```python
from build123d import *

# Parameters (mm, degrees)
ESQUISSE2_R             = 7
BOSS_EXTRU_2_DEPTH      = 22
ENL_V_MAT_EXTRU_1_DEPTH = 19
ESQUISSE5_R             = 5.5
ENL_V_MAT_EXTRU_2_DEPTH = 105.177732746
ENL_V_START             = -36
ENL_V_MAT_EXTRU_3_DEPTH = 24
COQUE1_START            = 3
COQUE1_DEPTH            = 19
COQUE1_START_2          = 15
COQUE1_2_OUTLINE_R      = 6.5
COQUE1_2_DEPTH          = 7
ENL_V_MAT_EXTRU_4_REACH = 106.178
ESQUISSE16_R            = 6.5
ENL_V_START_2           = -13
ENL_V_MAT_EXTRU_5_DEPTH = 13


# Read off the part's stored shape, not the designer's step: Coque1
with BuildPart() as part:
    # Esquisse2 → Boss.-Extru.2 (new, symmetric)
    with BuildSketch(Plane.XY):
        with BuildLine():
            Line((51.296980053, -19), (57, -19))
            Line((57, -19), (86, 15))
            Line((86, 15), (86, 34))
            Line((86, 34), (81, 39))
            Line((81, 39), (57, 39))
            ThreePointArc((57, 39), (48.490791592, 29.99016727), (36.246410316, 28.077357637))
            Line((36.246410316, 28.077357637), (14, 32))
            Line((14, 32), (7, 32))
            Line((7, 32), (0, 25))
            Line((0, 25), (0, 7))
            Line((0, 7), (7, 0))
            Line((7, 0), (39.575538911, 0))
            ThreePointArc((39.575538911, 0), (42.840774692, -1.213413768), (44.521177653, -4.264705882))
            ThreePointArc((44.521177653, -4.264705882), (46.858007856, -12.115672061), (51.296980053, -19))
        make_face()
        with Locations((14, 14)):
            Circle(ESQUISSE2_R, mode=Mode.SUBTRACT)
    extrude(amount=BOSS_EXTRU_2_DEPTH, both=True)

    # Esquisse4 → Enlèv. mat.-Extru.1 (cut)
    with BuildSketch(Plane.XY.offset(22)):
        Polygon((34, 32), (0, 32), (0, -19), (86, -19), (86, 0), (34, 0), align=None)
    extrude(amount=-ENL_V_MAT_EXTRU_1_DEPTH, mode=Mode.SUBTRACT)

    # Esquisse5 → Enlèv. mat.-Extru.2 (cut, through all)
    with BuildSketch(Plane.XY.offset(22)):
        with Locations((72, 25)):
            Circle(ESQUISSE5_R)
    extrude(amount=-ENL_V_MAT_EXTRU_2_DEPTH, mode=Mode.SUBTRACT)

    # Esquisse14 → Enlèv. mat.-Extru.3 (cut)
    with BuildSketch(Plane(origin=(0, 0, -22), x_dir=(-1, 0, 0), z_dir=(0, 0, -1)).offset(ENL_V_START)):
        with BuildLine():
            Line((-75.764705882, 3), (-86, 15))
            Line((-86, 15), (-86, 34))
            Line((-86, 34), (-81, 39))
            Line((-81, 39), (-57, 39))
            ThreePointArc((-57, 39), (-53.002548038, 33.285750119), (-47.224051208, 29.381745985))
            ThreePointArc((-47.224051208, 29.381745985), (-58.169717695, 12.59414375), (-75.764705882, 3))
        make_face()
    extrude(amount=ENL_V_MAT_EXTRU_3_DEPTH, mode=Mode.SUBTRACT)

    # Coque1 outline → Coque1 (cut)
    with BuildSketch(Plane.XY.offset(COQUE1_START)):
        with BuildLine():
            Line((72.744476296, 1), (73.986847747, 2.456573425))
            ThreePointArc((73.986847747, 2.456573425), (57.296143365, 12.041008897), (46.63326541, 28.064243583))
            ThreePointArc((46.63326541, 28.064243583), (41.418086005, 26.871182604), (36.072762138, 27.092549884))
            Line((36.072762138, 27.092549884), (35, 27.281706793))
            Line((35, 27.281706793), (35, 1))
            Line((35, 1), (72.744476296, 1))
        make_face()
    extrude(amount=COQUE1_DEPTH, mode=Mode.SUBTRACT)

    # Coque1 2 outline → Coque1 2 (cut)
    with BuildSketch(Plane.XY.offset(COQUE1_START_2)):
        with BuildLine():
            Line((73.986847747, 2.456573425), (85, 15.368545033))
            Line((85, 15.368545033), (85, 33.585786438))
            Line((85, 33.585786438), (80.585786438, 38))
            Line((80.585786438, 38), (57.631958739, 38))
            ThreePointArc((57.631958739, 38), (53.079347815, 31.984103338), (46.63326541, 28.064243583))
            ThreePointArc((46.63326541, 28.064243583), (57.296143365, 12.041008897), (73.986847747, 2.456573425))
        make_face()
        with Locations((72, 25)):
            Circle(COQUE1_2_OUTLINE_R, mode=Mode.SUBTRACT)
    extrude(amount=COQUE1_2_DEPTH, mode=Mode.SUBTRACT)

    # Esquisse16 → Enlèv. mat.-Extru.4 (cut, up to next)
    with BuildSketch(Plane.XY.offset(22), mode=Mode.PRIVATE) as enl_v_mat_extru_4_sk1:
        with Locations(Location((72, 25, 0), (0, 0, 180))):
            Circle(ESQUISSE16_R)
    enl_v_mat_extru_4_tool1 = extrude(enl_v_mat_extru_4_sk1.sketch, amount=-ENL_V_MAT_EXTRU_4_REACH, mode=Mode.PRIVATE) & part.part
    add(enl_v_mat_extru_4_tool1.solids().sort_by_distance((72, 25, 22))[0], mode=Mode.SUBTRACT)

    # Esquisse17 → Enlèv. mat.-Extru.5 (cut)
    with BuildSketch(Plane.XY.offset(3).offset(ENL_V_START_2)):
        with BuildLine():
            Line((72.744476296, 1), (73.986847747, 2.456573425))
            ThreePointArc((73.986847747, 2.456573425), (57.296143365, 12.041008897), (46.63326541, 28.064243583))
            ThreePointArc((46.63326541, 28.064243583), (41.418086005, 26.871182604), (36.072762138, 27.092549884))
            Line((36.072762138, 27.092549884), (35, 27.281706793))
            Line((35, 27.281706793), (35, 1))
            Line((35, 1), (72.744476296, 1))
        make_face()
    extrude(amount=ENL_V_MAT_EXTRU_5_DEPTH, mode=Mode.SUBTRACT)


solid = part.part
```
For this review, take the finished solid that the model builds, in its own axes (mm). A direction names the side the tool comes from. Round coordinates to 2 decimals unless told otherwise and drop trailing zeros. Write each loop counter-clockwise with the first axis right and the second up, starting at its lowest first coordinate (ties: lowest second). Pieces come first, ordered by that corner, then holes. Notation, with made-up numbers: (44, 80.25) - (68, 80.25) arc R24 cw to (68, 113.25) - close; hole circle Ø3 at (44, 88). An arc over 180 degrees is marked (long way). Answer as CSV lines item,"result". Start each with the question number.
(1) For line 1 (Y direction, x = 72, z = 14.4); line 2 (Z direction, x = 42, y = 11); line 3 (Y direction, x = 14, z = -9), list the stretches that pass through material, from the lowest coordinate up.
(2) Add section C-C, the plane z = -6. State the section outline as (x, y) points.
(3) Machinability: for faces 4 (the cylindrical face through (65.8, 23.05, 14.51)), 5 (the flat face through (56, -7, 3)), 6 (the flat face through (11, 32, -9)), which of the approach directions +Z, -Z, +X, -X, +Y, -Y give a long, thin tool a straight path to every point of the face, cutting with its end or side? Answer none if there is none.
(4) For pin 1 (1.5 mm diameter, centred on x = 65.5, y = 24, fed in from +Z); pin 2 (3.5 mm diameter, centred on x = 65.5, z = 19.5, fed in from -Y); pin 3 (13 mm diameter, centred on y = 12, z = 3, fed in from +X); pin 4 (10.5 mm diameter, centred on x = 72, y = 25, fed in from +Z), all flat-tipped, find the tip position at first contact; note any pin that passes through.
(5) Add section D-D, the plane x = 63. State the section outline as (y, z) points.
(6) Add section B-B, the plane y = 8. State the section outline as (x, z) points, plus the area to 3 significant figures.
(7) Add section A-A, the plane z = 9.5. State the section outline as (x, y) points, plus the area to 3 significant figures.
(8) Mouldability with a two-part tool opening along X and no side actions: class faces 1 (the cylindrical face through (57.495, 11.856, 2.325)), 2 (the flat face through (46, 28, 22)), 3 (the cylindrical face through (42.8, -1.18, -9.32)) as +X half, -X half, draft (parallel to the pull), parting line (faces both ways), or undercut.
From the geometry:
1,line 1,"y = 0 to 1, 3.1 to 18.5, 31.5 to 39"
1,line 2,"z = -22 to -10"
1,line 3,"y = 0 to 7, 21 to 32"
2,outline,"(0, 7) - (7, 0) - (39.58, 0) arc R5 cw to (44.52, -4.26) arc R29 ccw to (51.3, -19) - (57, -19) - (75.76, 3) arc R41 cw to (47.22, 29.38) arc R19.15 cw to (36.25, 28.08) - (14, 32) - (7, 32) - (0, 25) - close; hole circle Ø14 at (14, 14); hole (35, 1) - (72.74, 1) - (73.99, 2.46) arc R42 cw to (46.63, 28.06) arc R20.15 cw to (36.07, 27.09) - (35, 27.28) - close"
3,face 4,"+Z"
3,face 5,"+Z, +X, -X, -Y"
3,face 6,"+Z, -Z, -X, +Y"
4,pin 1,"stops at z = 15"
4,pin 2,"stops at y = 0"
4,pin 3,"stops at x = 68.77"
4,pin 4,"passes through"
5,outline,"(-11.97, -22) - (39, -22) - (39, -10) - (8.76, -10) - (8.76, 14) - (39, 14) - (39, 22) - (38, 22) - (38, 15) - (7.56, 15) - (7.56, -10) - (1, -10) - (1, 22) - (0, 22) - (0, 3) - (-11.97, 3) - close"
6,outline,"(0, -22) - (10.39, -22) - (10.39, 3) - (0, 3) - close; (17.61, -22) - (80.03, -22) - (80.03, -10) - (64.16, -10) - (64.16, 14) - (80.03, 14) - (80.03, 22) - (78.72, 22) - (78.72, 15) - (62.34, 15) - (62.34, -10) - (35, -10) - (35, 22) - (34, 22) - (34, 3) - (17.61, 3) - close"
6,area,"1,320 mm²"
7,outline,"(34, 0) - (73.21, 0) - (75.76, 3) arc R41 cw to (47.22, 29.38) arc R19.15 cw to (36.25, 28.08) - (34, 28.47) - close; hole (35, 1) - (72.74, 1) - (73.99, 2.46) arc R42 cw to (46.63, 28.06) arc R20.15 cw to (36.07, 27.09) - (35, 27.28) - close"
7,area,"121 mm²"
8,face 1,"undercut"
8,face 2,"draft"
8,face 3,"-X half"
